from build123d import *

# Parameters (mm, degrees)
F1_DEPTH  = 6
F2_R      = 3
F3_DEPTH  = 0.5
F4_R      = 3
F5_DEPTH  = 0.5
F6_R      = 2.99999
F7_R      = 2.99999
F9_DEPTH  = 1.1
F11_DEPTH = 1.2
F12_R     = 2.99999
F14_DEPTH = 13.4
F16_DEPTH = 0.1
F18_DEPTH = 0.1


# Not quite as in the source:
# - a fillet or chamfer is up to 0.001 mm smaller than in the source, because OpenCascade refuses the exact size


with BuildPart() as f1:
    # F0 (on Top) → F1 (new body)
    with BuildSketch(Plane.XY):
        with BuildLine():
            Line((-3.15, 8.1), (-3.15, 10.1734949747))
            ThreePointArc((-3.15, 10.1734949747), (-5.6194604457, 9.046776459), (-7.7238904562, 7.3323949854))
            ThreePointArc((-7.7238904562, 7.3323949854), (0, -10.65), (7.7238904562, 7.3323949854))
            ThreePointArc((7.7238904562, 7.3323949854), (5.6194604457, 9.046776459), (3.15, 10.1734949747))
            Line((3.15, 10.1734949747), (3.15, 8.1))
            Line((3.15, 8.1), (0, 8.1))
            Line((0, 8.1), (-3.15, 8.1))
        make_face()
        with BuildLine():
            ThreePointArc((3.15, 0), (-2.2273863607, -2.2273863607), (0, 3.15))
            ThreePointArc((0, 3.15), (2.2273863607, 2.2273863607), (3.15, 0))
        make_face(mode=Mode.SUBTRACT)
        with BuildLine():
            ThreePointArc((-7.7238904562, 7.3323949854), (-5.6194604457, 9.046776459), (-3.15, 10.1734949747))
            Line((-3.15, 10.1734949747), (-3.15, 23.35))
            Line((-3.15, 23.35), (-9.6377339195, 19.5871143267))
            Line((-9.6377339195, 19.5871143267), (-9.6377339195, 10.6575252249))
            ThreePointArc((-9.6377339195, 10.6575252249), (-8.1670066914, 9.2906908645), (-7.7238904562, 7.3323949854))
        make_face()
        with BuildLine():
            ThreePointArc((3.15, 10.1734949747), (5.6194604457, 9.046776459), (7.7238904562, 7.3323949854))
            ThreePointArc((7.7238904562, 7.3323949854), (8.1670066914, 9.2906908645), (9.6377339195, 10.6575252249))
            Line((9.6377339195, 10.6575252249), (9.6377339195, 19.5871143267))
            Line((9.6377339195, 19.5871143267), (3.15, 23.35))
            Line((3.15, 23.35), (3.15, 10.1734949747))
        make_face()
    extrude(amount=F1_DEPTH)

    # F2 (on face) → F3 (join)
    with BuildSketch(Plane.YZ.offset(-3.15)):
        with Locations((18.85, 3)):
            Circle(F2_R)
    extrude(amount=F3_DEPTH)

    # F4 (on face) → F5 (join)
    with BuildSketch(Plane(origin=(3.15, 0, 0), x_dir=(0, -1, 0), z_dir=(-1, 0, 0))):
        with Locations((-18.85, 3)):
            Circle(F4_R)
    extrude(amount=F5_DEPTH)

    # F6 (radius 3 in the source; OpenCascade refuses exactly that, so slightly less here)
    f6_edges = [f1.edges().sort_by_distance(p)[0] for p in [
        (-6.393867, 21.468557, 0),
        (-6.393867, 21.468557, 6),
    ]]
    fillet(f6_edges, radius=F6_R)

    # F7 (radius 3 in the source; OpenCascade refuses exactly that, so slightly less here)
    f7_edges = [f1.edges().sort_by_distance(p)[0] for p in [
        (6.393867, 21.468557, 0),
        (6.393867, 21.468557, 6),
    ]]
    fillet(f7_edges, radius=F7_R)

    # F8 (on face) → F9 (cut)
    with BuildSketch(Plane.XY.offset(6)):
        Polygon((-0.5410675658, -4.1934514275), (-0.2322952287, -4.1934514275), (-1.4496098506, -6.0194233604), (-2.6669244725, -4.1934514275), (-2.3, -4.1934514275), (-2.3, -3.9827399887), (-3.5, -3.9827399887), (-3.5, -4.1934514275), (-3.1341812573, -4.1934514275), (-2.8992197012, -4.5418942706), (-1.6819050793, -6.3678662034), (-3.0600394749, -8.4350677969), (-3.1399389263, -8.5422809794), (-3.5, -8.5422809794), (-3.5, -8.7529924182), (-2.3, -8.7529924182), (-2.3, -8.5422809794), (-2.6669244725, -8.5422809794), (-1.4496098506, -6.7163090465), (-0.2322952287, -8.5422809794), (-0.5410675658, -8.5422809794), (-0.5410675658, -8.7529924182), (0.5013382179, -8.7529924182), (0.5013382179, -8.5422809794), (0.2322952287, -8.5422809794), (1.4496098506, -6.7163090465), (2.6669244725, -8.5422809794), (2.3810260464, -8.5422809794), (2.3810260464, -8.7529924182), (3.4986780956, -8.7529924182), (3.5, -8.5422809794), (3.1424169429, -8.5422809794), (3.0600394749, -8.4350677969), (1.6819050793, -6.3678662034), (2.8992197012, -4.5418942706), (3.1315149299, -4.1934514275), (3.3579636365, -4.1934514275), (3.5, -4.1934514275), (3.4986780956, -3.9827399887), (2.3810260464, -3.9827399887), (2.3810260464, -4.1934514275), (2.6669244725, -4.1934514275), (1.4496098506, -6.0194233604), (0.1581401168, -4.1934514275), (0.5013382179, -4.1934514275), (0.5013382179, -3.9827399887), (-0.5410675658, -3.9827399887), align=None)
        Polygon((-1.2173146219, -6.3678662034), (0, -4.5418942706), (1.2173146219, -6.3678662034), (0, -8.1938381363), align=None, mode=Mode.SUBTRACT)
    extrude(amount=-F9_DEPTH, mode=Mode.SUBTRACT)

    # F10 (on face) → F11 (cut)
    with BuildSketch(Plane(origin=(0, 0, 0), x_dir=(1, 0, 0), z_dir=(0, 0, -1))):
        Polygon((-0.6402181378, 8.4924687258), (-0.3314458007, 8.4924687258), (-1.5487604226, 6.6664967929), (-2.7660750445, 8.4924687258), (-2.399150572, 8.4924687258), (-2.399150572, 8.7031801646), (-3.599150572, 8.7031801646), (-3.599150572, 8.4924687258), (-3.2333318293, 8.4924687258), (-2.9983702732, 8.1440258827), (-1.7810556513, 6.3180539499), (-3.1591900469, 4.2508523564), (-3.2390894983, 4.1436391739), (-3.599150572, 4.1436391739), (-3.599150572, 3.9329277351), (-2.399150572, 3.9329277351), (-2.399150572, 4.1436391739), (-2.7660750445, 4.1436391739), (-1.5487604226, 5.9696111068), (-0.3314458007, 4.1436391739), (-0.6402181378, 4.1436391739), (-0.6402181378, 3.9329277351), (0.4021876459, 3.9329277351), (0.4021876459, 4.1436391739), (0.1331446567, 4.1436391739), (1.3504592786, 5.9696111068), (2.5677739006, 4.1436391739), (2.2818754744, 4.1436391739), (2.2818754744, 3.9329277351), (3.3995275237, 3.9329277351), (3.400849428, 4.1436391739), (3.0432663709, 4.1436391739), (2.960888903, 4.2508523564), (1.5827545073, 6.3180539499), (2.8000691293, 8.1440258827), (3.032364358, 8.4924687258), (3.2588130645, 8.4924687258), (3.400849428, 8.4924687258), (3.3995275237, 8.7031801646), (2.2818754744, 8.7031801646), (2.2818754744, 8.4924687258), (2.5677739006, 8.4924687258), (1.3504592786, 6.6664967929), (0.0589895449, 8.4924687258), (0.4021876459, 8.4924687258), (0.4021876459, 8.7031801646), (-0.6402181378, 8.7031801646), align=None)
        Polygon((-1.3164651939, 6.3180539499), (-0.099150572, 8.1440258827), (1.1181640499, 6.3180539499), (-0.099150572, 4.492082017), align=None, mode=Mode.SUBTRACT)
    extrude(amount=-F11_DEPTH, mode=Mode.SUBTRACT)

    # F12 (radius 3 in the source; OpenCascade refuses exactly that, so slightly less here)
    f12_edges = [f1.edges().sort_by_distance(p)[0] for p in [
        (0, 8.1, 0),
        (0, 8.1, 6),
    ]]
    fillet(f12_edges, radius=F12_R)

    # F13 (on Top) → F14 (cut)
    with BuildSketch(Plane.XY):
        Polygon((-3.4496616572, 8.1000812352), (-3.1200703233, 8.1000812352), (-3.1314746011, 15.4313463718), (-3.4496616572, 15.4313463718), align=None)
        Polygon((3.1499122269, 8.1000812352), (3.4496616572, 8.1000812352), (3.4496616572, 15.4313463718), (3.1314746011, 15.4313463718), align=None)
    extrude(amount=F14_DEPTH, mode=Mode.SUBTRACT)

    # F15 (on face) → F16 (cut)
    with BuildSketch(Plane(origin=(0, 0, 0), x_dir=(1, 0, 0), z_dir=(0, 0, -1))):
        with BuildLine():
            Line((9.7270584918, -4.3366845744), (9.7615409984, -4.3366845744))
            ThreePointArc((9.7615409984, -4.3366845744), (0, 10.6815034411), (-9.7615409984, -4.3366845744))
            Line((-9.7615409984, -4.3366845744), (-9.7270584918, -4.3366845744))
            Line((-9.7270584918, -4.3366845744), (9.7270584918, -4.3366845744))
        make_face()
    extrude(amount=-F16_DEPTH, mode=Mode.SUBTRACT)

    # F17 (on face) → F18 (cut)
    with BuildSketch(Plane.XY.offset(6)):
        with BuildLine():
            Line((9.646881219, 4.4377580388), (-9.6813637257, 4.4377580388))
            ThreePointArc((-9.6813637257, 4.4377580388), (0, -10.65), (9.6813637257, 4.4377580388))
            Line((9.6813637257, 4.4377580388), (9.646881219, 4.4377580388))
        make_face()
    extrude(amount=-F18_DEPTH, mode=Mode.SUBTRACT)


solid = f1.part
Geometry: final body of the model. Coordinates: model frame, mm. A direction names the side the tool comes from. Coordinates: 2 decimals unless noted, no trailing zeros. Order: outer loops, then holes, each group sorted by start corner. A loop starts at its lowest first (then second) coordinate and runs counter-clockwise, first axis right, second up. Notation, with made-up numbers: (50.25, 86.25) - (93.25, 86.25) arc R17 ccw to (93.25, 92.25) - close; hole circle Ø7 at (87, -12.75). An arc over 180 degrees is marked (long way). Use one line per item in the form item = value.
1) Section A-A (y = 12). Return loops of the section in (x, z).
Solutions:
outline = (-9.64, 0) - (-3.45, 0) - (-3.45, 6) - (-9.64, 6) - close; (3.45, 0) - (9.64, 0) - (9.64, 6) - (3.45, 6) - close
2) Section B-B (z = 1.6). Return loops of the section in (x, y).
Solutions:
outline = (-9.64, 10.66) arc R3.4 cw to (-7.72, 7.33) arc R10.65 ccw (long way) to (7.72, 7.33) arc R3.4 cw to (9.64, 10.66) - (9.64, 19.19) - (3.15, 22.95) - (3.15, 21.5) - (2.65, 21.5) - (2.65, 16.2) - (3.15, 16.2) - (3.15, 15.43) - (3.45, 15.43) - (3.45, 8.1) - (3.15, 8.1) - (3.15, 7.75) - (-3.15, 7.75) - (-3.15, 8.1) - (-3.45, 8.1) - (-3.45, 15.43) - (-3.15, 15.43) - (-3.15, 16.2) - (-2.65, 16.2) - (-2.65, 21.5) - (-3.15, 21.5) - (-3.15, 22.95) - (-9.64, 19.19) - close; hole circle Ø6.3 at (0, 0)
3) Pin query (flat end, axial travel): pin 1 (1.8 mm diameter, centred on y = 19.5, z = 3, fed in from +X); pin 2 (1.2 mm diameter, centred on x = 3, z = 1, fed in from -Y); pin 3 (3 mm diameter, centred on y = 8.5, z = 5.5, fed in from -X). Return the tip coordinate at first contact, or that it passes through.
Solutions:
pin_1 = 9.64
pin_2 = -10.38
pin_3 = -8.71
4) Mould query, pull axis Y, two halves, no side actions, for faces 5 (the face through (6.7, 20.3, 5.1)), 6 (the face through (-1.2, -5.8, 1.2)), 7 (the face through (2, -3, 5.9)). Classes: +Y half, -Y half, draft (parallel to the pull), parting line (faces both ways), or undercut.
Solutions:
face_5 = +Y half
face_6 = undercut
face_7 = draft
5) Ray query, L1, parallel to X at y = 16.5, z = 3.15; L2, parallel to X at y = 15, z = 2.95; L3, parallel to X at y = -8.5, z = 4.95. Return the intervals inside material, ascending.
Solutions:
L1 = -9.64 to -2.65, 2.65 to 9.64
L2 = -9.64 to -3.45, 3.45 to 9.64
L3 = -6.42 to -3.11, -2.64 to -0.26, 0.26 to 2.64, 3.11 to 6.42
6) Set-up query: faces 1 (the face through (-2.9, 21.71, 3.9)), 2 (the face through (8.153, 9.266, 2.958)), 3 (the face through (-2.3, -5.44, 5.41)), 4 (the face through (-0.04, 7.2, 0.86)). Return all of +Z, -Z, +X, -X, +Y, -Y with unobstructed straight access to the full face (end or side cutting, diameter ignored); none if empty.
Solutions:
face_1 = none
face_2 = +Z, -Z, +X
face_3 = +Z
face_4 = -Z
